```python
from build123d import *

# Parameters (mm, degrees)
EXTRUDE_1_DEPTH     = 50
SHELL_1_T           = -4
SKETCH_2_R          = 3
SKETCH_2_R_2        = 3.425496854
EXTRUDE_2_DEPTH     = 3
SKETCH_4_R          = 1.60000254
CUT_EXTRUDE_2_DEPTH = 4
SKETCH_7_R          = 2.25
CUT_EXTRUDE_4_DEPTH = 5
SKETCH_8_W          = 5
SKETCH_8_H          = 40
CUT_EXTRUDE_5_DEPTH = 144
SKETCH_9_W          = 5
SKETCH_9_H          = 40
CUT_EXTRUDE_6_DEPTH = 28
EXTRUDE_START       = -10
SKETCH_5_W          = 10
SKETCH_5_H          = 10
EXTRUDE_4_DEPTH     = 10
SKETCH_6_R          = 2.75
CUT_EXTRUDE_3_DEPTH = 4
FILLET_1_R          = 5
SKETCH_13_W         = 20.178165971
SKETCH_13_H         = 15.738969457
SKETCH_13_W_2       = 16.343899967
SKETCH_13_H_2       = 8.864106926
EXTRUDE_6_DEPTH     = 4
SKETCH_14_W         = 16.343899967
SKETCH_14_H         = 8.864106926
CUT_EXTRUDE_8_DEPTH = 10
FILLET_2_R          = 1


with BuildPart() as part:
    # 草图1 → 凸台-拉伸1 (new body)
    with BuildSketch(Plane(origin=(0, 0, 0), x_dir=(1, 0, 0), z_dir=(0, 1, 0))):
        with BuildLine():
            Line((-50, -50), (-50, 50))
            Line((-50, 50), (50, 50))
            Line((50, 50), (50, -50))
            ThreePointArc((50, -50), (0, -100), (-50, -50))
        make_face()
    extrude(amount=EXTRUDE_1_DEPTH)

    # 抽壳1
    shell_1_openings = [part.faces().sort_by_distance(p)[0] for p in [
        (0, 50, 20.082075005),
    ]]
    offset(amount=SHELL_1_T, openings=shell_1_openings, kind=Kind.INTERSECTION)

    # 草图2 → 凸台-拉伸2 (add)
    with BuildSketch(Plane(origin=(0, 4, 0), x_dir=(1, 0, 0), z_dir=(0, 1, 0))):
        with Locations(Location((35.632314962, -14.68949484, 0), (0, 0, 270))):
            Circle(SKETCH_2_R)
        with Locations(Location((35.760604874, 35.310439638, 0), (0, 0, 270))):
            Circle(SKETCH_2_R)
        with Locations(Location((-35, 36, 0), (0, 0, 270))):
            Circle(SKETCH_2_R_2)
        with Locations(Location((-34.367594322, -14.509888959, 0), (0, 0, 270))):
            Circle(SKETCH_2_R)
    extrude(amount=EXTRUDE_2_DEPTH)

    # 草图4 → 切除-拉伸2 (cut)
    with BuildSketch(Plane(origin=(0, 7, 0), x_dir=(1, 0, 0), z_dir=(0, 1, 0))):
        with Locations(Location((-34.367594322, -14.509888959, 0), (0, 0, 270))):
            Circle(SKETCH_4_R)
        with Locations(Location((-35, 36, 0), (0, 0, 270))):
            Circle(SKETCH_4_R)
        with Locations(Location((35.760604874, 35.310439638, 0), (0, 0, 270))):
            Circle(SKETCH_4_R)
        with Locations(Location((35.632314962, -14.68949484, 0), (0, 0, 270))):
            Circle(SKETCH_4_R)
    extrude(amount=-CUT_EXTRUDE_2_DEPTH, mode=Mode.SUBTRACT)

    # 草图7 → 切除-拉伸4 (cut)
    with BuildSketch(Plane(origin=(0, 4, 0), x_dir=(1, 0, 0), z_dir=(0, 1, 0))):
        with Locations(Location((-38, 26, 0), (0, 0, 270))):
            Circle(SKETCH_7_R)
        with Locations(Location((38, 26, 0), (0, 0, 270))):
            Circle(SKETCH_7_R)
        with Locations(Location((38, -26, 0), (0, 0, 270))):
            Circle(SKETCH_7_R)
        with Locations(Location((-38, -26, 0), (0, 0, 270))):
            Circle(SKETCH_7_R)
    extrude(amount=-CUT_EXTRUDE_4_DEPTH, mode=Mode.SUBTRACT)

    # 草图8 → 切除-拉伸5 (cut)
    with BuildSketch(Plane(origin=(50, 0, 0), x_dir=(0, 0, -1), z_dir=(1, 0, 0))):
        with Locations((-42.5, 25)):
            Rectangle(SKETCH_8_W, SKETCH_8_H)
        with Locations((-32.5, 25)):
            Rectangle(SKETCH_8_W, SKETCH_8_H)
        with Locations((-22.5, 25)):
            Rectangle(SKETCH_8_W, SKETCH_8_H)
        with Locations((-12.5, 25)):
            Rectangle(SKETCH_8_W, SKETCH_8_H)
        with Locations((-2.5, 25)):
            Rectangle(SKETCH_8_W, SKETCH_8_H)
        with Locations((7.5, 25)):
            Rectangle(SKETCH_8_W, SKETCH_8_H)
        with Locations((17.5, 25)):
            Rectangle(SKETCH_8_W, SKETCH_8_H)
        with Locations((27.5, 25)):
            Rectangle(SKETCH_8_W, SKETCH_8_H)
        with Locations((37.5, 25)):
            Rectangle(SKETCH_8_W, SKETCH_8_H)
    extrude(amount=-CUT_EXTRUDE_5_DEPTH, mode=Mode.SUBTRACT)

    # 草图9 → 切除-拉伸6 (cut)
    with BuildSketch(Plane(origin=(0, 0, -50), x_dir=(-1, 0, 0), z_dir=(0, 0, -1))):
        with Locations((0, 25)):
            Rectangle(SKETCH_9_W, SKETCH_9_H)
        with Locations((10, 25)):
            Rectangle(SKETCH_9_W, SKETCH_9_H)
        with Locations((20, 25)):
            Rectangle(SKETCH_9_W, SKETCH_9_H)
        with Locations((30, 25)):
            Rectangle(SKETCH_9_W, SKETCH_9_H)
        with Locations((40, 25)):
            Rectangle(SKETCH_9_W, SKETCH_9_H)
        with Locations((-10, 25)):
            Rectangle(SKETCH_9_W, SKETCH_9_H)
        with Locations((-20, 25)):
            Rectangle(SKETCH_9_W, SKETCH_9_H)
        with Locations((-30, 25)):
            Rectangle(SKETCH_9_W, SKETCH_9_H)
        with Locations((-40, 25)):
            Rectangle(SKETCH_9_W, SKETCH_9_H)
    extrude(amount=-CUT_EXTRUDE_6_DEPTH, mode=Mode.SUBTRACT)

    # 草图5 → 凸台-拉伸4 (add)
    with BuildSketch(Plane(origin=(0, 50, 0), x_dir=(1, 0, 0), z_dir=(0, 1, 0)).offset(EXTRUDE_START)):
        with Locations((-41, 41)):
            Rectangle(SKETCH_5_W, SKETCH_5_H)
        with Locations((41, 41)):
            Rectangle(SKETCH_5_W, SKETCH_5_H)
        with BuildLine():
            Line((34.871191548, -80), (-34.871191548, -80))
            ThreePointArc((-34.871191548, -80), (0, -96), (34.871191548, -80))
        make_face()
    extrude(amount=EXTRUDE_4_DEPTH)

    # 草图6 → 切除-拉伸3 (cut)
    with BuildSketch(Plane(origin=(0, 50, 0), x_dir=(1, 0, 0), z_dir=(0, 1, 0))):
        with Locations(Location((43, 43, 0), (0, 0, 270))):
            Circle(SKETCH_6_R)
        with Locations(Location((0, -90, 0), (0, 0, 270))):
            Circle(SKETCH_6_R)
        with Locations(Location((-43, 43, 0), (0, 0, 90))):
            Circle(SKETCH_6_R)
    extrude(amount=-CUT_EXTRUDE_3_DEPTH, mode=Mode.SUBTRACT)

    # 圆角1
    fillet_1_edges = [part.edges().sort_by_distance(p)[0] for p in [
        (-50, 25, -50),
        (50, 25, -50),
    ]]
    fillet(fillet_1_edges, radius=FILLET_1_R)

    # 草图13 → 凸台-拉伸6 (add)
    with BuildSketch(Plane(origin=(0, 0, -50), x_dir=(-1, 0, 0), z_dir=(0, 0, -1))):
        with Locations((24.507779854, 11.808957997)):
            Rectangle(SKETCH_13_W, SKETCH_13_H)
        with Locations((23.205413146, 12.661389703)):
            Rectangle(SKETCH_13_W_2, SKETCH_13_H_2, mode=Mode.SUBTRACT)
    extrude(amount=-EXTRUDE_6_DEPTH)

    # 草图14 → 切除-拉伸8 (cut)
    with BuildSketch(Plane(origin=(0, 0, -50), x_dir=(-1, 0, 0), z_dir=(0, 0, -1))):
        with Locations((23.205413146, 12.661389703)):
            Rectangle(SKETCH_14_W, SKETCH_14_H)
    extrude(amount=-CUT_EXTRUDE_8_DEPTH, mode=Mode.SUBTRACT)

    # 圆角2
    fillet_2_edges = [part.edges().sort_by_distance(p)[0] for p in [
        (-31.37736313, 17.093443166, -48),
        (-31.37736313, 8.22933624, -48),
        (-15.033463163, 17.093443166, -48),
        (-15.033463163, 8.22933624, -48),
    ]]
    fillet(fillet_2_edges, radius=FILLET_2_R)


solid = part.part
```
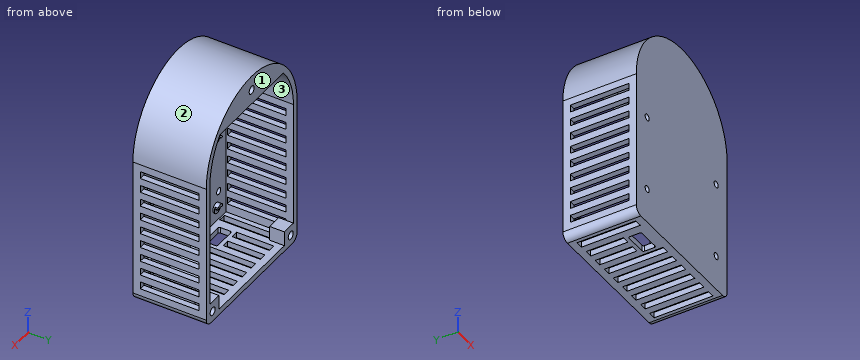
Input: part model. Units: mm. Frame: model coordinates. Face numbers are marked on the shaded views. Round coordinates to 2 decimals unless told otherwise and drop trailing zeros. Loops run counter-clockwise (first coordinate to the right, second up) from the corner with the lowest first, then second, coordinate; pieces in that order, holes last. Notation, with made-up numbers: M 52,-27.75 L 89,-27.75 A12 cw 89,-14.75 Z; hole C 56.25,-40 d3. An arc over 180 degrees is marked long. Answer in a Markdown table with one row per item. Add a question column.
1. Ray query, probe 1 along X at (y, z) = (47.1, -43); probe 2 along X at (y, z) = (2, 26); probe 3 along Y at (x, z) = (28, 84). Return the intervals inside material, ascending.
2. Mould query, pull axis Z, two halves, no side actions, for the marked faces 1, 2 and 3. Classes: released by +Z, released by -Z, zero draft, split by the parting line, or undercut.
3. Section B-B (x = 0). Output: boundary loops of the cut face in (y, z), and give its area (3 significant figures).
4. Section A-A (z = 43). Output: boundary loops of the cut face in (x, y).
5. Contact query for flat-ended pins moving along their axis: pin 1 (2 mm diameter, centred on x = 48.5, y = 33, fed in from -Z); pin 2 (2 mm diameter, centred on y = 12.5, z = -48.5, fed in from -X); pin 3 (1.2 mm diameter, centred on x = -48.5, y = 19, fed in from -Z). Output: stop coordinate, or through.
6. Section C-C (y = 26). Give the number of separate pieces and of enclosed holes in the cut face, and give its area (3 significant figures).
Values follow:
| question | item | result |
|---|---|---|
| 1 | probe 1 | -50 to -45.75, -40.25 to -36, 36 to 40.25, 45.75 to 50 |
| 1 | probe 2 | -50 to -40.25, -35.75 to 35.75, 40.25 to 50 |
| 1 | probe 3 | 0 to 4, 40 to 50 |
| 2 | face 1 | zero draft |
| 2 | face 2 | released by +Z |
| 2 | face 3 | undercut |
| 3 | outline | M 0,-50 L 5,-50 L 5,-46 L 4,-46 L 4,96 L 40,96 L 40,80 L 50,80 L 50,87.25 L 46,87.25 L 46,92.75 L 50,92.75 L 50,100 L 0,100 Z; M 45,-50 L 50,-50 L 50,-46 L 45,-46 Z |
| 3 | area | 946 mm^2 |
| 4 | outline | M -50,0 L 50,0 L 50,5 L 46,5 L 46,4 L -46,4 L -46,5 L -50,5 Z; M -50,45 L -46,45 L -46,50 L -50,50 Z; M 46,45 L 50,45 L 50,50 L 46,50 Z |
| 5 | pin 1 | z = -49.33 |
| 5 | pin 2 | x = -49.33 |
| 5 | pin 3 | z = -49.07 |
| 6 | separate pieces | 27 |
| 6 | enclosed holes | 0 |
| 6 | area | 1,220 mm^2 |
